The figure shows three views and two pictorial views of one solid part (mm, origin at its lowest corner). Answer the questions. A direction names the side the tool comes from. Round coordinates to 2 decimals unless told otherwise and drop trailing zeros. Write each loop counter-clockwise with the first axis right and the second up, starting at its lowest first coordinate (ties: lowest second). Pieces come first, ordered by that corner, then holes. Notation, with made-up numbers: (22.25, 79) -> (70.25, 79) arc R19 cw to (70.25, 104) -> close; hole circle Ø10 at (-16, -3.75). An arc over 180 degrees is marked (long way). One line per item, written item: value.
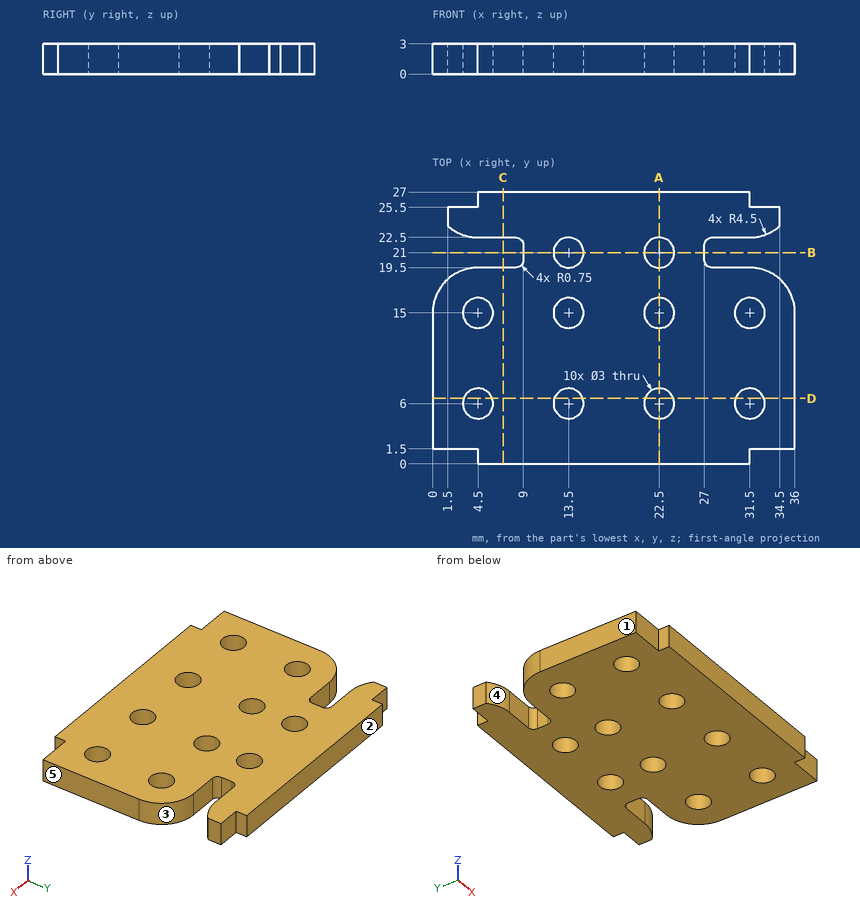
(1) For a pull along Y with two mould halves and no side action, classify the marked faces 1, 2 and 3 as pulls with the +Y half, pulls with the -Y half, needs draft (parallel to the pull), parting line crosses it, or undercut.
Reported:
face 1: needs draft
face 2: pulls with the +Y half
face 3: undercut
(2) Find section A-A on x = 22.5. Give the vertices of the cut face in (y, z).
Reported:
outline: (0, 0) -> (4.5, 0) -> (4.5, 3) -> (0, 3) -> close; (7.5, 0) -> (13.5, 0) -> (13.5, 3) -> (7.5, 3) -> close; (16.5, 0) -> (19.5, 0) -> (19.5, 3) -> (16.5, 3) -> close; (22.5, 0) -> (27, 0) -> (27, 3) -> (22.5, 3) -> close
(3) Find section C-C on x = 7. Give the vertices of the cut face in (y, z).
Reported:
outline: (0, 0) -> (19.5, 0) -> (19.5, 3) -> (0, 3) -> close; (22.5, 0) -> (27, 0) -> (27, 3) -> (22.5, 3) -> close
(4) A tool of negligible diameter and unlimited length cuts with its end or side. For the marked faces 4 and 5, from which of +Z, -Z, +X, -X, +Y, -Y can it reach the whole face along a straight path? Write none if from no direction.
Reported:
face 4: +Z, -Z, -X
face 5: +Z, -Z, +X, +Y, -Y
(5) Find section D-D on y = 6.5. Give the vertices of the cut face in (x, z).
Reported:
outline: (0, 0) -> (3.09, 0) -> (3.09, 3) -> (0, 3) -> close; (5.91, 0) -> (12.09, 0) -> (12.09, 3) -> (5.91, 3) -> close; (14.91, 0) -> (21.09, 0) -> (21.09, 3) -> (14.91, 3) -> close; (23.91, 0) -> (30.09, 0) -> (30.09, 3) -> (23.91, 3) -> close; (32.91, 0) -> (36, 0) -> (36, 3) -> (32.91, 3) -> close
(6) Consider probe 1 along X at (y, z) = (15, 0.75); probe 2 along Y at (x, z) = (13.5, 0.7); probe 3 along Y at (x, z) = (5.5, 1.5). Determine where each line is inside the solid, lowest interval first.
Reported:
probe 1: x = 0 to 3, 6 to 12, 15 to 21, 24 to 30, 33 to 36
probe 2: y = 0 to 4.5, 7.5 to 13.5, 16.5 to 19.5, 22.5 to 27
probe 3: y = 0 to 4.88, 7.12 to 13.88, 16.12 to 19.5, 22.5 to 27
(7) Flat-ended cylindrical pins translate along their axes: pin 1 Ø4 at (x, y) = (13.5, 6) entering from -Z; pin 2 Ø1.6 at (y, z) = (20.5, 1) entering from +X; pin 3 Ø1.5 at (x, z) = (1.5, 2) entering from -Y; pin 4 Ø0.9 at (y, z) = (25, 2) entering from -X. Find the tip coordinate at first contact, or state that the pin passes through.
Reported:
pin 1: stops at z = 0
pin 2: stops at x = 27.24
pin 3: stops at y = 1.5
pin 4: stops at x = 1.5
(8) Find section B-B on y = 21. Give the vertices of the cut face in (x, z), plus the area to 3 significant figures.
Reported:
outline: (9, 0) -> (12, 0) -> (12, 3) -> (9, 3) -> close; (15, 0) -> (21, 0) -> (21, 3) -> (15, 3) -> close; (24, 0) -> (27, 0) -> (27, 3) -> (24, 3) -> close
area: 36.0 mm2
